Build history of the part. All positions in model axes, mm. Face numbers are marked on the shaded views. A direction names the side the tool comes from. Give positions to 0.01 mm unless a question says otherwise; leave off trailing zeros. Write each loop counter-clockwise with the first axis right and the second up, starting at its lowest first coordinate (ties: lowest second). Pieces come first, ordered by that corner, then holes. Notation, with made-up numbers: (78, 37.25) -> (110, 37.25) arc R23 cw to (110, 68.25) -> close; hole circle Ø2 at (77.25, 6.5). An arc over 180 degrees is marked (long way). One line per question, with ' | ' between items. Start each with the question number.
(1) Band-saw the part on C-C, the plane y = 0. Give the cut face in (x, z), and give its area (3 significant figures).
(2) Band-saw the part on A-A, the plane y = -22. Give the cut face in (x, z).
(3) Pull direction Y, two halves, no side cores. Call the marked faces 1, 2 and 3: released by +Y, released by -Y, zero draft, split by the parting line, or undercut.
(4) Band-saw the part on D-D, the plane y = 27. Give the cut face in (x, z), and give its area (3 significant figures).
(5) Band-saw the part on B-B, the plane x = 2.5. Give the cut face in (y, z), and give its area (3 significant figures).
(6) Drill centre lines: probe 1 along Y at (x, z) = (0, 5.5); probe 2 along X at (y, z) = (-15.5, 3.5); probe 3 along X at (y, z) = (30, 5). Where is each one in solid material? Low to high. Write a range as from..to.
(7) Tool access for the marked faces 4 and 5: list every direction of +Z, -Z, +X, -X, +Y, -Y with a clear straight run to the whole face (end or side of a thin tool).
(8) Pin check, flat tips, straight feed: P1, Ø4, axis at y = 35.5, z = 5, coming from the -X side; P2, Ø1, axis at y = -12.5, z = 3, coming from the -X side; P3, Ø3, axis at x = 22.5, z = 5.5, coming from the +Y side. Stop position of each tip, or through.
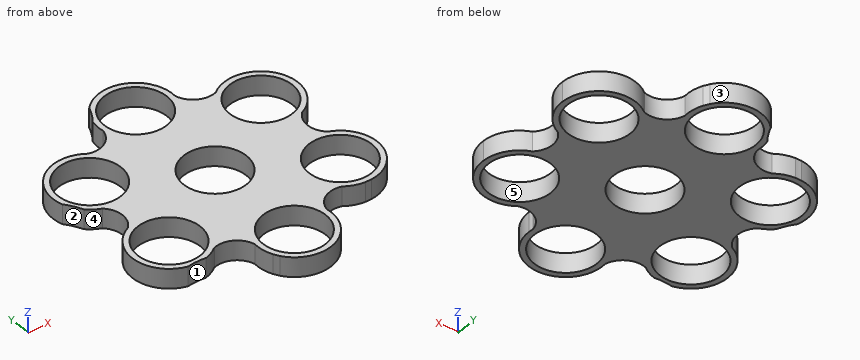
from build123d import *

# Parameters (mm, degrees)
F0_R     = 11.2
F0_R_2   = 13.2
F1_DEPTH = 7


with BuildPart() as f1:
    # F0 (on Top) → F1 (new body)
    with BuildSketch(Plane.XY):
        with BuildLine():
            ThreePointArc((-36.21903, 5.78652), (-19.634866, 11.382994), (-23.185572, 28.522057))
            ThreePointArc((-23.185572, 28.522057), (-26.275542, 30.239878), (-29.710626, 31.075951))
            ThreePointArc((-29.710626, 31.075951), (-30.764801, 31.077003), (-31.817763, 31.127599))
            ThreePointArc((-31.817763, 31.127599), (-41.802797, 25.655223), (-43.814174, 14.447985))
            ThreePointArc((-43.814174, 14.447985), (-41.972925, 11.717586), (-40.55145, 8.746949))
            ThreePointArc((-40.55145, 8.746949), (-38.533827, 7.049286), (-36.21903, 5.78652))
        make_face()
        with Locations((-31.086612, 17.947864)):
            Circle(F0_R, mode=Mode.SUBTRACT)
        with BuildLine():
            ThreePointArc((-9.394765, 45.168181), (-10.838735, 42.208413), (-12.700645, 39.492061))
            ThreePointArc((-12.700645, 39.492061), (-13.162052, 36.895916), (-13.098242, 34.25986))
            ThreePointArc((-13.098242, 34.25986), (0.040529, 22.69579), (13.10804, 34.340323))
            ThreePointArc((13.10804, 34.340323), (13.050731, 37.875226), (12.05725, 41.268132))
            ThreePointArc((12.05725, 41.268132), (11.531073, 42.181601), (11.04841, 43.11879))
            ThreePointArc((11.04841, 43.11879), (1.316676, 49.029895), (-9.394765, 45.168181))
        make_face()
        with Locations((0, 35.895728)):
            Circle(F0_R, mode=Mode.SUBTRACT)
        with BuildLine():
            ThreePointArc((44.286612, 17.947864), (36.964159, 29.767104), (23.120788, 28.47334))
            ThreePointArc((23.120788, 28.47334), (19.675395, 11.312796), (36.293612, 5.818266))
            ThreePointArc((36.293612, 5.818266), (39.326273, 7.635348), (41.767875, 10.192181))
            ThreePointArc((41.767875, 10.192181), (42.295874, 11.104598), (42.866173, 11.991191))
            ThreePointArc((42.866173, 11.991191), (43.926593, 14.886018), (44.286612, 17.947864))
        make_face()
        with Locations((31.086612, 17.947864)):
            Circle(F0_R, mode=Mode.SUBTRACT)
        with BuildLine():
            ThreePointArc((13.10804, 34.340323), (0.040529, 22.69579), (-13.098242, 34.25986))
            ThreePointArc((-13.098242, 34.25986), (-16.865441, 29.14687), (-23.185572, 28.522057))
            ThreePointArc((-23.185572, 28.522057), (-19.634866, 11.382994), (-36.21903, 5.78652))
            ThreePointArc((-36.21903, 5.78652), (-33.67465, -0.032465), (-36.293612, -5.818266))
            ThreePointArc((-36.293612, -5.818266), (-19.675395, -11.312796), (-23.120788, -28.47334))
            ThreePointArc((-23.120788, -28.47334), (-16.80921, -29.179335), (-13.10804, -34.340323))
            ThreePointArc((-13.10804, -34.340323), (-0.040529, -22.69579), (13.098242, -34.25986))
            ThreePointArc((13.098242, -34.25986), (16.865441, -29.14687), (23.185572, -28.522057))
            ThreePointArc((23.185572, -28.522057), (19.634866, -11.382994), (36.21903, -5.78652))
            ThreePointArc((36.21903, -5.78652), (33.67465, 0.032465), (36.293612, 5.818266))
            ThreePointArc((36.293612, 5.818266), (19.675395, 11.312796), (23.120788, 28.47334))
            ThreePointArc((23.120788, 28.47334), (16.80921, 29.179335), (13.10804, 34.340323))
        make_face()
        Circle(F0_R_2, mode=Mode.SUBTRACT)
        with BuildLine():
            ThreePointArc((44.286612, -17.947864), (42.086337, -10.650875), (36.21903, -5.78652))
            ThreePointArc((36.21903, -5.78652), (19.634866, -11.382994), (23.185572, -28.522057))
            ThreePointArc((23.185572, -28.522057), (26.275542, -30.239878), (29.710626, -31.075951))
            ThreePointArc((29.710626, -31.075951), (30.764801, -31.077003), (31.817763, -31.127599))
            ThreePointArc((31.817763, -31.127599), (40.675438, -27.01949), (44.286612, -17.947864))
        make_face()
        with Locations((31.086612, -17.947864)):
            Circle(F0_R, mode=Mode.SUBTRACT)
        with BuildLine():
            ThreePointArc((13.098242, -34.25986), (-0.040529, -22.69579), (-13.10804, -34.340323))
            ThreePointArc((-13.10804, -34.340323), (-13.050731, -37.875226), (-12.05725, -41.268132))
            ThreePointArc((-12.05725, -41.268132), (-11.531073, -42.181601), (-11.04841, -43.11879))
            ThreePointArc((-11.04841, -43.11879), (3.768354, -48.5464), (13.2, -35.895728))
            ThreePointArc((13.2, -35.895728), (13.174536, -35.076213), (13.098242, -34.25986))
        make_face()
        with Locations((0, -35.895728)):
            Circle(F0_R, mode=Mode.SUBTRACT)
        with BuildLine():
            ThreePointArc((-23.120788, -28.47334), (-19.675395, -11.312796), (-36.293612, -5.818266))
            ThreePointArc((-36.293612, -5.818266), (-39.326273, -7.635348), (-41.767875, -10.192181))
            ThreePointArc((-41.767875, -10.192181), (-42.295874, -11.104598), (-42.866173, -11.991191))
            ThreePointArc((-42.866173, -11.991191), (-43.119473, -23.374673), (-34.419409, -30.720196))
            ThreePointArc((-34.419409, -30.720196), (-31.13419, -30.490827), (-27.850805, -30.745112))
            ThreePointArc((-27.850805, -30.745112), (-25.371774, -29.84663), (-23.120788, -28.47334))
        make_face()
        with Locations((-31.086612, -17.947864)):
            Circle(F0_R, mode=Mode.SUBTRACT)
        Circle(F0_R_2)
        Circle(F0_R, mode=Mode.SUBTRACT)
    extrude(amount=F1_DEPTH)


solid = f1.part
Results:
1) outline: (-33.67, 0) -> (-11.2, 0) -> (-11.2, 7) -> (-33.67, 7) -> close; (11.2, 0) -> (33.67, 0) -> (33.67, 7) -> (11.2, 7) -> close | area: 315 mm²
2) outline: (-43.65, 0) -> (-41.53, 0) -> (-41.53, 7) -> (-43.65, 7) -> close; (-20.65, 0) -> (20.65, 0) -> (20.65, 7) -> (-20.65, 7) -> close; (41.53, 0) -> (43.65, 0) -> (43.65, 7) -> (41.53, 7) -> close
3) face 1: released by -Y | face 2: undercut | face 3: released by +Y
4) outline: (-40.69, 0) -> (-37.68, 0) -> (-37.68, 7) -> (-40.69, 7) -> close; (-24.49, 0) -> (-6.8, 0) -> (-6.8, 7) -> (-24.49, 7) -> close; (6.8, 0) -> (24.49, 0) -> (24.49, 7) -> (6.8, 7) -> close; (37.68, 0) -> (40.69, 0) -> (40.69, 7) -> (37.68, 7) -> close | area: 290 mm²
5) outline: (-48.86, 0) -> (-46.81, 0) -> (-46.81, 7) -> (-48.86, 7) -> close; (-24.98, 0) -> (-10.92, 0) -> (-10.92, 7) -> (-24.98, 7) -> close; (10.92, 0) -> (24.98, 0) -> (24.98, 7) -> (10.92, 7) -> close; (46.81, 0) -> (48.86, 0) -> (48.86, 7) -> (46.81, 7) -> close | area: 225 mm²
6) probe 1: y = -49.1..-47.1, -24.7..-11.2, 11.2..24.7, 47.1..49.1 | probe 2: x = -44.06..-42.02, -20.16..20.16, 42.02..44.06 | probe 3: x = -36.47..-25.7, -15.65..-9.52, 9.52..15.66, 25.7..36.47
7) face 4: +Z, -Z, -X | face 5: +Z, -Z
8) P1: stops at x = -13.31 | P2: stops at x = -43.32 | P3: stops at y = 29.08
